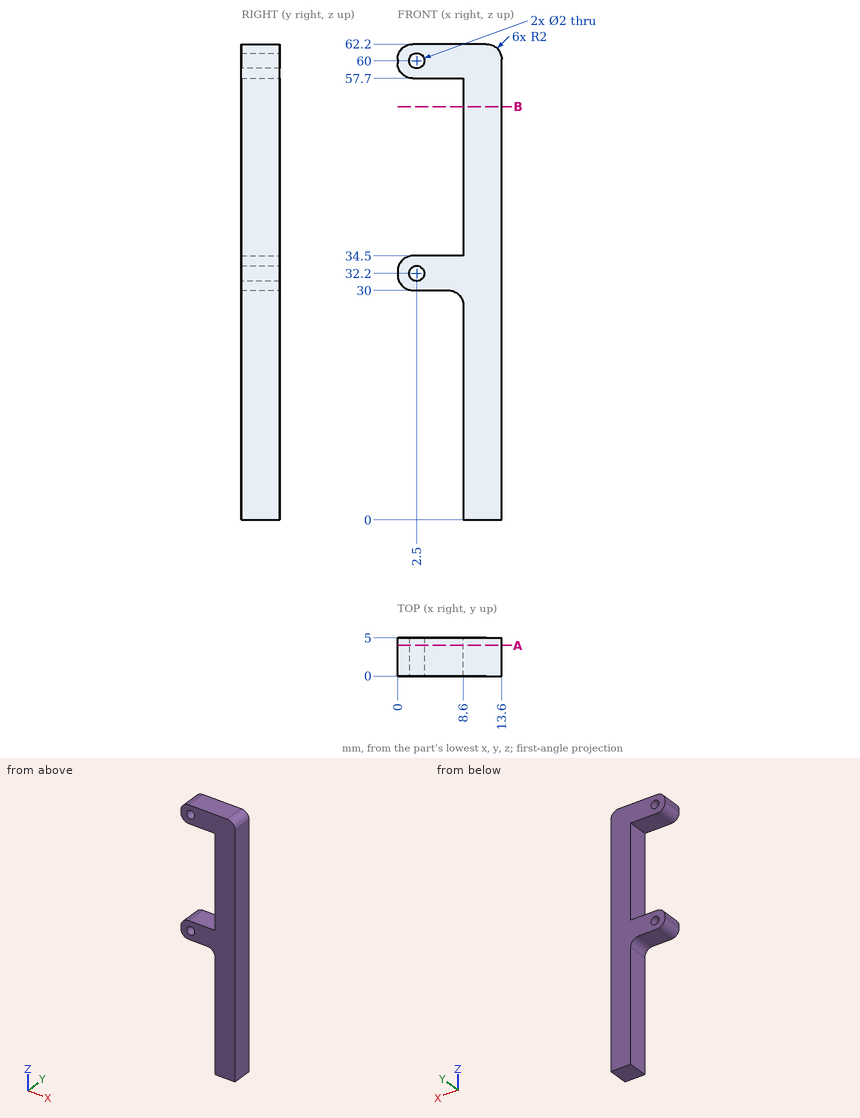
For this review, use the dimensioned drawing (mm, ordinates from the lowest corner) and the shaded views. Coordinates: 2 decimals unless noted, no trailing zeros. Write each loop counter-clockwise with the first axis right and the second up, starting at its lowest first coordinate (ties: lowest second). Pieces come first, ordered by that corner, then holes. Notation, with made-up numbers: (32.25, -17.75) - (90.25, -17.75) arc R24 ccw to (90.25, -6.75) - close; hole circle Ø11 at (-0.5, 55). An arc over 180 degrees is marked (long way). Answer in a Markdown table with one row per item. Add a question column.
Q1. Consider section A-A on y = 4. Give the boundary of the cut face in (x, z).
Q2. To check wall thickness, follow line 1 along Z through (x, y) = (2.25, 4.6); line 2 along X through (y, z) = (3.15, 32.2); line 3 along Z through (x, y) = (1.75, 2.35). State the ranges of each line that lie inside material, in increasing order. Write a range as from..to.
Q3. Clearance check with flat-ended pins moving along their axes: pin 1 (1 mm diameter, centred on y = 4, z = 28, fed in from -X); pin 2 (1.2 mm diameter, centred on x = 2.5, z = 60, fed in from -Y); pin 3 (1.5 mm diameter, centred on y = 1.5, z = 41, fed in from -X); pin 4 (1.5 mm diameter, centred on x = 6, y = 3.5, fed in from -Z). State where each tip first meets the part, or that it passes through.
Q4. Consider section B-B on z = 54. Give the boundary of the cut face in (x, y), then the cut area to 3 significant figures.
Answers below:
| question | item | result |
|---|---|---|
| 1 | outline | (0, 32) arc R2 ccw to (2, 30) - (6.6, 30) arc R2 cw to (8.6, 28) - (8.6, 0) - (13.6, 0) - (13.6, 60.2) arc R2 ccw to (11.6, 62.2) - (2, 62.2) arc R2 ccw to (0, 60.2) - (0, 59.7) arc R2 ccw to (2, 57.7) - (8.6, 57.7) - (8.6, 34.5) - (2, 34.5) arc R2 ccw to (0, 32.5) - close; hole circle Ø2 at (2.5, 32.2); hole circle Ø2 at (2.5, 60) |
| 2 | line 1 | 30..31.23, 33.17..34.5, 57.7..59.03, 60.97..62.2 |
| 2 | line 2 | 0..1.5, 3.5..13.6 |
| 2 | line 3 | 30.02..31.54, 32.86..34.48, 57.72..59.34, 60.66..62.18 |
| 3 | pin 1 | x = 8.54 |
| 3 | pin 2 | through |
| 3 | pin 3 | x = 8.6 |
| 3 | pin 4 | z = 29.99 |
| 4 | outline | (8.6, 0) - (13.6, 0) - (13.6, 5) - (8.6, 5) - close |
| 4 | area | 25.0 mm² |
